Verification items for the finished model (mm, model axes). A direction names the side the tool comes from. Give positions to 0.01 mm unless a question says otherwise; leave off trailing zeros. Order: outer loops, then holes, each group sorted by start corner. A loop starts at its lowest first (then second) coordinate and runs counter-clockwise, first axis right, second up. Notation, with made-up numbers: M -20.75,54 L -7.75,54 A20 cw -7.75,92 Z; hole C 31.5,-40 d5. An arc over 180 degrees is marked long. Answer as a JSON object with one key per item and string values.
```python
from build123d import *

# Parameters (mm, degrees)
ESQUISSE1_R             = 28
BOSS_EXTRU_1_DEPTH      = 5
ESQUISSE2_R             = 10
BOSS_EXTRU_2_DEPTH      = 6
ESQUISSE3_R             = 2.5
ENL_V_MAT_EXTRU_1_DEPTH = 42.097445176
ESQUISSE4_R             = 2


with BuildPart() as part:
    # Esquisse1 → Boss.-Extru.1 (new body)
    with BuildSketch(Plane.XY):
        Circle(ESQUISSE1_R)
    extrude(amount=BOSS_EXTRU_1_DEPTH)

    # Esquisse2 → Boss.-Extru.2 (add)
    with BuildSketch(Plane.XY.offset(5)):
        Circle(ESQUISSE2_R)
    extrude(amount=BOSS_EXTRU_2_DEPTH)

    # Esquisse3 → Enlèv. mat.-Extru.1 (cut, through all)
    with BuildSketch(Plane.XY.offset(11)):
        Circle(ESQUISSE3_R)
    extrude(amount=-ENL_V_MAT_EXTRU_1_DEPTH, mode=Mode.SUBTRACT)

    # Esquisse4 → Enlèvement de matière-Révolution1 (revolve, cut)
    with BuildSketch(Plane(origin=(0, 0, 0), x_dir=(0, 0, -1), z_dir=(1, 0, 0)), mode=Mode.PRIVATE) as enl_vement_de_mati_re_r_volution1_sk:
        with Locations((-2.5, 28)):
            Circle(ESQUISSE4_R)
    revolve(enl_vement_de_mati_re_r_volution1_sk.sketch.rotate(Axis((0, 0, 0), (0, 0, 1)), 90), axis=Axis((0, 0, 0), (0, 0, 1)), mode=Mode.SUBTRACT)


solid = part.part
```
Q1. Section check A-A on x = 0. Record the cut outline in (y, z), then the cut area to 3 significant figures.
Resolved:
{"outline": "M -28,0 L -2.5,0 L -2.5,11 L -10,11 L -10,5 L -28,5 L -28,4.5 A2 cw -28,0.5 Z; M 2.5,0 L 28,0 L 28,0.5 A2 cw 28,4.5 L 28,5 L 10,5 L 10,11 L 2.5,11 Z", "area": "332 mm²"}
Q2. Material ranges on L1, parallel to Y at x = 0, z = 6.25; L2, parallel to Z at x = -17, y = 8.5; L3, parallel to Z at x = 26, y = -6.5, recorded low to high.
Resolved:
{"L1": "y = -10 to -2.5, 2.5 to 10", "L2": "z = 0 to 5", "L3": "z = 0 to 0.9, 4.1 to 5"}
Q3. Section check C-C on z = 9.5. Record the cut outline in (x, y), then the cut area to 3 significant figures.
Resolved:
{"outline": "C 0,0 d20; hole C 0,0 d5", "area": "295 mm²"}
Q4. Gauge pin test, flat ends, axial feed: pin 1 Ø3 at (x, z) = (-15.5, 5) entering from +Y; pin 2 Ø5 at (y, z) = (13.5, 5) entering from -X; pin 3 Ø2 at (y, z) = (-16, 5) entering from -X. Record the tip position at first contact, or that the pin passes through.
Resolved:
{"pin 1": "stops at y = 24.25", "pin 2": "stops at x = -25.75", "pin 3": "stops at x = -23.64"}
Q5. Tool access check on faces 1 (the face through (0, -12, 5)), 2 (the face through (6, 0, 0)). Record the directions out of +Z, -Z, +X, -X, +Y, -Y that give a thin tool (end or side, any length) a straight path to the whole face; none if there is none.
Resolved:
{"face 1": "+Z", "face 2": "-Z, +X, -X, +Y, -Y"}
Q6. Release check for a two-part mould opening along X. For faces 3 (the face through (2, -2, 11)), 4 (the face through (25.865, -10.724, 0.246)), 5 (the face through (-0.54, -2.44, 5.58)) record: +X half, -X half, draft (parallel to the pull), parting line (faces both ways), or undercut.
Resolved:
{"face 3": "draft", "face 4": "parting line", "face 5": "undercut"}
